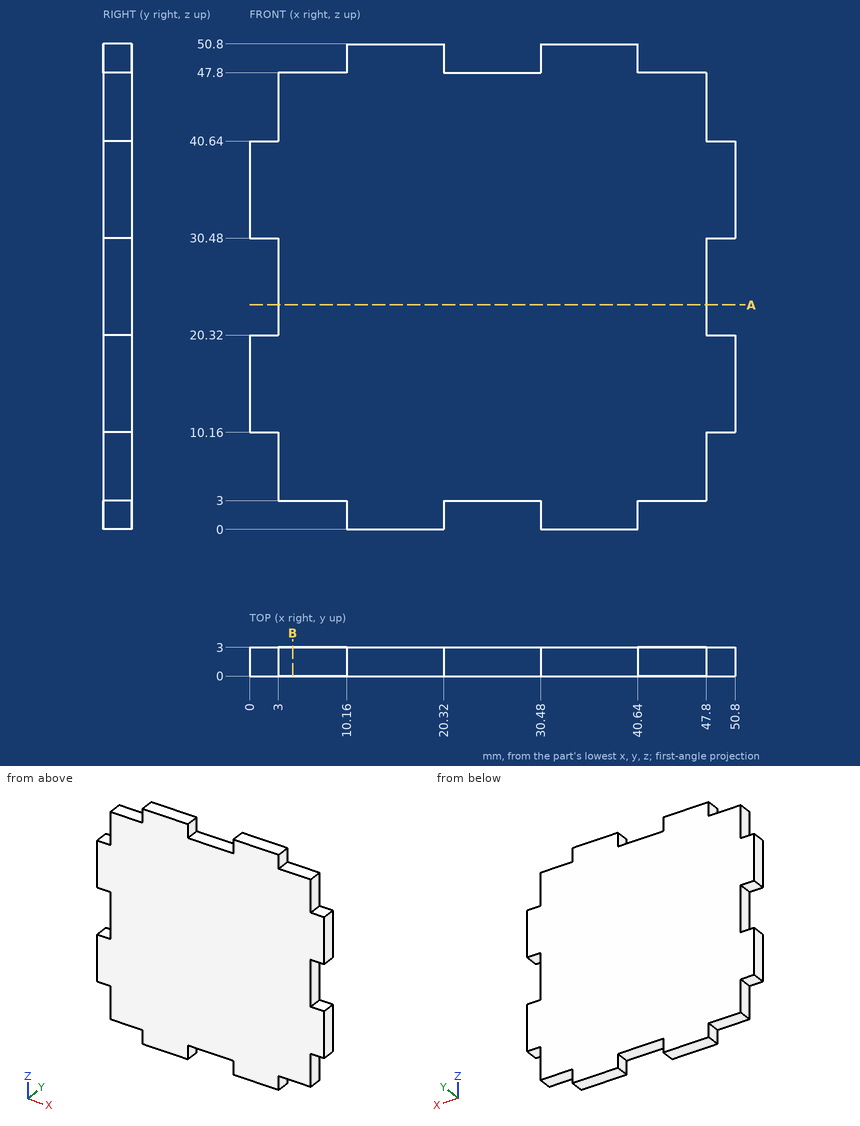
Here's the drawing with two shaded views (mm, measured from the low corner). I have some questions. Coordinates: 2 decimals unless noted, no trailing zeros. Loops run counter-clockwise (first coordinate to the right, second up) from the corner with the lowest first, then second, coordinate; pieces in that order, holes last. Notation, with made-up numbers: M 25,-25 L 73,-25 A20 cw 73,-10 Z; hole C -25.75,0 d11. An arc over 180 degrees is marked long. Put each result on its own line as item: value. Start each with the question number.
(1) Imagine slicing it at A-A on z = 23.5. List the corners of the cut face in (x, y) for me.
(2) Imagine slicing it at B-B on x = 4.5. List the corners of the cut face in (y, z) for me.
(3) Will these pins go through, and if not, where does the flat tip stop? pin 1 Ø0.9 at (y, z) = (1.5, 1.5) entering from +X; pin 2 Ø1.5 at (x, y) = (43, 1) entering from -Z; pin 3 Ø1.5 at (x, y) = (26.5, 1) entering from +Z.
(4) I need wall thicknesses on probe 1 along X at (y, z) = (1, 24); probe 2 along X at (y, z) = (2.75, 48). Which ranges of each line are inside material? Lowest first, please.
Worked answers:
1. outline: M 3,0 L 47.8,0 L 47.8,3 L 3,3 Z
2. outline: M 0,3 L 3,3 L 3,47.8 L 0,47.8 Z
3. pin 1: stops at x = 40.64
3. pin 2: stops at z = 3
3. pin 3: stops at z = 47.8
4. probe 1: x = 3 to 47.8
4. probe 2: x = 10.16 to 20.32, 30.48 to 40.64
